Build history of the part. All positions in model axes, mm. Give positions to 0.01 mm unless a question says otherwise; leave off trailing zeros. Write each loop counter-clockwise with the first axis right and the second up, starting at its lowest first coordinate (ties: lowest second). Pieces come first, ordered by that corner, then holes. Notation, with made-up numbers: (36, -19) -> (62, -19) arc R10 ccw to (62, -5) -> close; hole circle Ø3 at (46, -16.5). An arc over 180 degrees is marked (long way). Put each result on its own line as item: value. Start each with the question number.
Item 1: Drill centre lines: line 1 along Z through (x, y) = (0, 21); line 2 along Z through (x, y) = (7, 13.5); line 3 along X through (y, z) = (24.75, 5). Where is each one in solid material? Low to high.
Item 2: Slice it at D-D, the plane y = 4. List the corners of the cut face in (x, z) (3 decimals).
Item 3: Slice it at C-C, the plane y = 18.75. List the corners of the cut face in (x, z) (3 decimals).
Item 4: Two-plate mould, pull along X, no slides. Class faces 1 (the cylindrical face through (21.199, 11.166, 6.676)), 2 (the cylindrical face through (-15.12, 15.1, -11.59)), 3 (the conical face through (-4.163, 4.926, -18.747)): pulls with the +X half, pulls with the -X half, needs draft (parallel to the pull), parting line crosses it, or undercut.
Item 5: Slice it at A-A, the plane z = 0. List the corners of the cut face in (x, y) (3 decimals), plus the area to 3 significant figures.
Item 6: Flat gauge pins, fed straight in: pin 1 Ø12 at (y, z) = (4.5, 13.5) entering from -X; pin 2 Ø5 at (x, y) = (-0.5, 17) entering from +Z (3 decimals); pin 3 Ø5 at (y, z) = (16.5, 6) entering from +X. Where does each tip first touch, or does it go through?
Item 7: Slice it at B-B, the plane x = 0. List the corners of the cut face in (y, z) (3 decimals), plus the area to 3 significant figures.
```python
from build123d import *

# Parameters (mm, degrees)
F0_R     = 22.225
F1_DEPTH = 25.4
F2_T     = -3.175


# Not quite as in the source:
# - a fillet or chamfer that OpenCascade refuses, or shapes differently, is made with other operations: its cross-section is extruded or revolved along the edge and cut away or added


with BuildPart() as f1:
    # F0 (on Front) → F1 (new body)
    with BuildSketch(Plane.XZ):
        Circle(F0_R)
    extrude(amount=-F1_DEPTH)

    # F2
    f2_openings = [f1.faces().sort_by_distance(p)[0] for p in [
        (0, 0, 0),
        (0, 25.4, 0),
    ]]
    offset(amount=F2_T, openings=f2_openings)

    # F3: chamfer of 5.08 on 1 edges, made by hand

    # F3_s1 → F3_t2 (revolve, cut)
    with BuildSketch(Plane.XY):
        Polygon((24.13, 0), (19.05, 5.08), (19.05, 0), align=None)
    revolve(axis=Axis((0, 0, 0), (0, -1, 0)), mode=Mode.SUBTRACT)

    # F4: fillet of radius 5.08 on 1 edges, made by hand

    # F4_s1 → F4_t2 (revolve, cut)
    with BuildSketch(Plane.XY):
        with BuildLine():
            ThreePointArc((22.225, 20.6907139607), (21.3571134838, 23.5305202921), (19.05, 25.4))
            Line((19.05, 25.4), (22.225, 25.4))
            Line((22.225, 25.4), (22.225, 20.6907139607))
        make_face()
    revolve(axis=Axis((0, 25.4, 0), (0, -1, 0)), mode=Mode.SUBTRACT)


solid = f1.part
```
Values follow:
1. line 1: -22.22 to -19.05, 19.05 to 22.22
1. line 2: -21.09 to -17.72, 17.72 to 21.09
1. line 3: -19.57 to -18.38, 18.38 to 19.57
2. outline: circle Ø44.45 at (0, 0); hole circle Ø40.26 at (0, 0)
3. outline: circle Ø44.45 at (0, 0); hole circle Ø38.1 at (0, 0)
4. face 1: parting line crosses it
4. face 2: undercut
4. face 3: undercut
5. outline: (-22.225, 1.905) -> (-19.05, 5.08) -> (-19.05, 25.4) arc R5.08 ccw to (-22.225, 20.691) -> close; (19.05, 5.08) -> (22.225, 1.905) -> (22.225, 20.691) arc R5.08 ccw to (19.05, 25.4) -> close
5. area: 131 mm2
6. pin 1: x = -20.92
6. pin 2: z = 22.225
6. pin 3: x = 21.95
7. outline: (1.905, -22.225) -> (20.691, -22.225) arc R5.08 ccw to (25.4, -19.05) -> (5.08, -19.05) -> close; (1.905, 22.225) -> (5.08, 19.05) -> (25.4, 19.05) arc R5.08 ccw to (20.691, 22.225) -> close
7. area: 131 mm2
